Design review of the part built by this model. Coordinates are the model's own, in mm. Coordinates: 2 decimals unless noted, no trailing zeros. Write each loop counter-clockwise with the first axis right and the second up, starting at its lowest first coordinate (ties: lowest second). Pieces come first, ordered by that corner, then holes. Notation, with made-up numbers: (-30.75, 2.5) - (14.25, 2.5) arc R24 ccw to (14.25, 25.5) - close; hole circle Ø11 at (-9, -10). An arc over 180 degrees is marked (long way). Use a Markdown table: item, result.
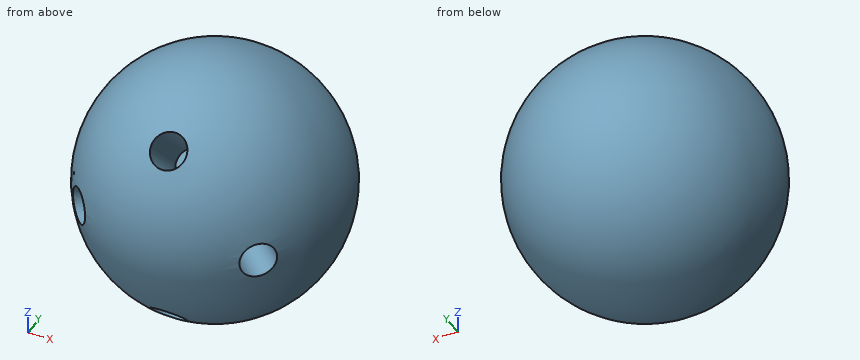
from build123d import *

# Parameters (mm, degrees)
F5_R            = 2.75
F6_DEPTH        = 11
F6_COPIES_COUNT = 4


# Not quite as in the source:
# - a pattern or mirror of a feature is missing from the dataset's text; its kind, count and spacing are read off the source's solid


with BuildPart() as f2:
    # F1 (on Front) → F2 (revolve)
    with BuildSketch(Plane.XZ):
        with BuildLine():
            ThreePointArc((0, 20), (-20, 0), (0, -20))
            Line((0, -20), (0, 20))
        make_face()
    revolve(axis=Axis((0, 0, 0), (0, 0, -1)))

    # F5 (on line) → F6 (cut)
    with BuildSketch(Plane(origin=(14.1421356237, -14.1421356237, 0), x_dir=(0.7071067812, 0.7071067812, 0), z_dir=(0.7071067812, -0.7071067812, 0))):
        Circle(F5_R)
    f6 = extrude(amount=-F6_DEPTH, mode=Mode.SUBTRACT)

    # F6_copies: F6 ×4 about axis
    f6_copies_axis = Axis((0, 0, 0), (0, 1, 0))
    for i in range(1, F6_COPIES_COUNT):
        add(f6.rotate(f6_copies_axis, i * 360 / F6_COPIES_COUNT), mode=Mode.SUBTRACT)


solid = f2.part
(1) For pin 1 (3 mm diameter, centred on x = -15.5, y = 15.5, fed in from +Z); pin 2 (3 mm diameter, centred on y = -2, z = 15.5, fed in from +X); pin 3 (4 mm diameter, centred on x = -6.5, z = 6.5, fed in from -Y); pin 4 (4 mm diameter, centred on x = -14, z = -1, fed in from -Y), all flat-tipped, find the tip position at first contact; note any pin that passes through.
Determined:
| item | result |
|---|---|
| pin 1 | through |
| pin 2 | x = 14.16 |
| pin 3 | y = -18.66 |
| pin 4 | y = -15.97 |
(2) Take a section at A-A on x = -1. Write out the cut boundary in (y, z), and give its area (3 significant figures).
Determined:
| item | result |
|---|---|
| outline | (-15.82, -12.2) - (-8.18, -4.55) - (-4.55, -8.18) - (-12.2, -15.82) arc R19.97 ccw (long way) to (-12.2, 15.82) - (-4.55, 8.18) - (-8.18, 4.55) - (-15.82, 12.2) arc R19.97 ccw to start |
| area | 1,140 mm2 |
(3) Take a section at C-C on y = 2. Write out the cut boundary in (x, z).
Determined:
| item | result |
|---|---|
| outline | circle Ø39.8 at (0, 0) |
(4) For L1, parallel to Y at x = 1, z = -5; L2, parallel to Y at x = -6, z = 1; L3, parallel to X at y = -6.5, z = 8, list the stretches that pass through material, from the lowest coordinate up. Write a range as from..to.
Determined:
| item | result |
|---|---|
| L1 | -19.34..-8.62, -7.73..19.34 |
| L2 | -19.05..-9.62, -6.73..19.05 |
| L3 | -17.14..-2.54, 2.54..17.14 |
(5) Take a section at B-B on y = 13. Write out the cut boundary in (x, z).
Determined:
| item | result |
|---|---|
| outline | circle Ø30.4 at (0, 0) |
